Part model, mm, in its own coordinate system. Coordinates: 2 decimals unless noted, no trailing zeros. Order: outer loops, then holes, each group sorted by start corner. A loop starts at its lowest first (then second) coordinate and runs counter-clockwise, first axis right, second up. Notation, with made-up numbers: M 80.25,85 L 116.25,85 A23 cw 116.25,94 Z; hole C -31,1 d4. An arc over 180 degrees is marked long. Answer in a Markdown table with one row per item. Add a question column.
Autodesk Inventor part; units mm, degrees
ref_plane "YZ Plane" through (0, 0, 0) normal (1, 0, 0) x (0, 1, 0)
ref_plane "XZ Plane" through (0, 0, 0) normal (0, 1, 0) x (-1, 0, 0)
ref_plane "XY Plane" through (0, 0, 0) normal (0, 0, 1) x (1, 0, 0)
sketch "Sketch1" plane through (0, 0, 0) normal (0, 0, 1) x (1, 0, 0)
  line L0 (0, 0) -> (45, 0)
  line L1 (45, 0) -> (45, 78.5)
  line L2 (45, 78.5) -> (0, 78.5)
  line L3 (0, 78.5) -> (0, 0)
  dimension "d0" = 45
  dimension "d1" = 78.5
extrude "Extrusion1" add sketch "Sketch1" along normal blind 3
sketch "Sketch2" plane through (0, 0, 3) normal (0, 0, 1) x (1, 0, 0)
  line L0 (0, 78.5) -> (-2, 78.5)
  line L1 (-2, 78.5) -> (-2, 80.5)
  line L2 (-2, 80.5) -> (0, 80.5)
  line L3 (0, 80.5) -> (0, 78.5)
  line L4 (45, 0) -> (47, 0)
  line L5 (47, 0) -> (47, -2)
  line L6 (47, -2) -> (45, -2)
  line L7 (45, -2) -> (45, 0)
  line L8 (-2, 80.5) -> (47, 80.5)
  line L9 (47, 80.5) -> (47, -2)
  line L10 (47, -2) -> (-2, -2)
  line L11 (-2, -2) -> (-2, 80.5)
  dimension "d4" = 2
  dimension "d5" = 2
  dimension "d6" = 2
  dimension "d7" = 2
extrude "Extrusion2" add sketch "Sketch2" along normal blind 3
properties part number "Transmitter Case Top"
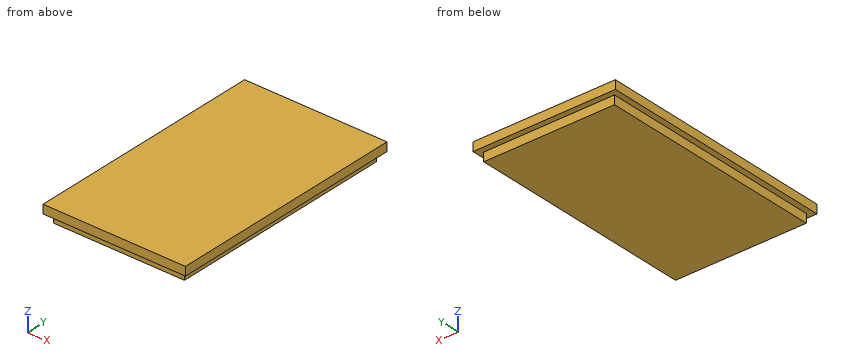
(1) Slice it at A-A (y = 53). List the corners of the cut face in (x, z).
(2) Drop flat-ended pins along their axis: P1, Ø1.5, axis at x = 30.5, z = 1.5, coming from the -Y side; P2, Ø0.9, axis at y = 20.5, z = 2, coming from the -X side; P3, Ø1.5, axis at x = 29.5, z = 1.5, coming from the +Y side. Give the stop position or say it passes through.
(3) Slice it at C-C (z = 1.4). List the corners of the cut face in (x, y), and give its area (3 significant figures).
(4) Wall check: line 1 (X direction, y = 43, z = 1.2); line 2 (Y direction, x = 38.5, z = 0.55). Give the ranges that are in metal, low to high.
(5) Slice it at B-B (x = 36). List the corners of the cut face in (y, z), and give its area (3 significant figures).
Computed:
| question | item | result |
|---|---|---|
| 1 | outline | M -2,3 L 0,3 L 0,0 L 45,0 L 45,3 L 47,3 L 47,6 L -2,6 Z |
| 2 | P1 | stops at y = 0 |
| 2 | P2 | stops at x = 0 |
| 2 | P3 | stops at y = 78.5 |
| 3 | outline | M 0,0 L 45,0 L 45,78.5 L 0,78.5 Z |
| 3 | area | 3,530 mm^2 |
| 4 | line 1 | x = 0 to 45 |
| 4 | line 2 | y = 0 to 78.5 |
| 5 | outline | M -2,3 L 0,3 L 0,0 L 78.5,0 L 78.5,3 L 80.5,3 L 80.5,6 L -2,6 Z |
| 5 | area | 483 mm^2 |
